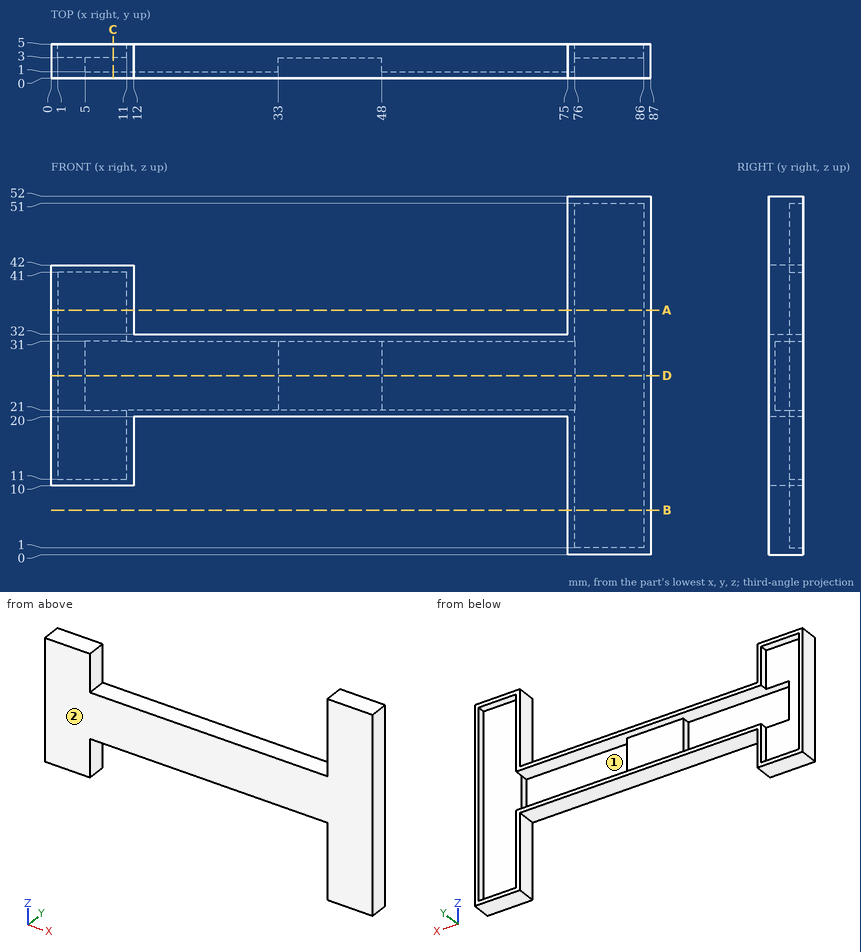
Check sheet for the drawn part. Datum: minimum x, y, z corner. Units: mm. Give positions to 0.01 mm unless a question says otherwise; leave off trailing zeros. Write each loop counter-clockwise with the first axis right and the second up, starting at its lowest first coordinate (ties: lowest second). Pieces come first, ordered by that corner, then holes. Notation, with made-up numbers: M 18,-17.5 L 32,-17.5 A30 ccw 32,18.5 Z; hole C 24,-22.75 d1. An arc over 180 degrees is marked long. One line per question, with ' | ' between items.
1) Section check C-C on x = 9. Enter the section's corners in (y, z).
Result:
outline: M 0,10 L 5,10 L 5,11 L 3,11 L 3,21 L 1,21 L 1,31 L 3,31 L 3,41 L 5,41 L 5,42 L 0,42 Z
2) Section check D-D on z = 26. Enter the section's corners in (x, y).
Result:
outline: M 0,0 L 87,0 L 87,5 L 86,5 L 86,3 L 76,3 L 76,1 L 48,1 L 48,3 L 33,3 L 33,1 L 5,1 L 5,3 L 1,3 L 1,5 L 0,5 Z
3) Gauge pin test, flat ends, axial feed: pin 1 Ø2.5 at (x, y) = (46.5, 3.5) entering from -Z; pin 2 Ø5 at (x, z) = (4, 18.5) entering from +Y. Record the tip position at first contact, or that the pin passes through.
Result:
pin 1: stops at z = 20 | pin 2: stops at y = 3
4) Section check A-A on z = 35.5. Enter the section's corners in (x, y), plus the area to 3 significant figures.
Result:
outline: M 0,0 L 12,0 L 12,5 L 11,5 L 11,3 L 1,3 L 1,5 L 0,5 Z; M 75,0 L 87,0 L 87,5 L 86,5 L 86,3 L 76,3 L 76,5 L 75,5 Z | area: 80.0 mm2
5) Section check B-B on z = 6.5. Enter the section's corners in (x, y).
Result:
outline: M 75,0 L 87,0 L 87,5 L 86,5 L 86,3 L 76,3 L 76,5 L 75,5 Z
6) Mould release check, pull along Z, two halves, no side actions. Record for the marked faces 1 and 2: released by +Z, released by -Z, zero draft, split by the parting line, or undercut.
Result:
face 1: undercut | face 2: zero draft
7) Thickness scan on line 1 along Z through (x, y) = (48, 3.4); line 2 along Z through (x, y) = (4.5, 4.6); line 3 along X through (y, z) = (0.55, 35.5). Record the ranges inside material, lowest first. Write a range as [from, to].
Result:
line 1: z = [20, 21], [31, 32] | line 2: z = [10, 11], [41, 42] | line 3: x = [0, 12], [75, 87]
